from build123d import *

# Parameters (mm, degrees)
F0_R      = 38.1
F1_DEPTH  = 123.825
F2_R      = 6.35
F1_FACE_R = 31.75
F3_DEPTH  = 114.3
F4_R      = 4.292472


with BuildPart() as f1:
    # F0 (on Front) → F1 (new body)
    with BuildSketch(Plane.XZ):
        Circle(F0_R)
    extrude(amount=F1_DEPTH)

    # F2
    f2_edges = [f1.edges().sort_by_distance(p)[0] for p in [
        (-38.1, -123.825, 0),
    ]]
    fillet(f2_edges, radius=F2_R)

    # F1_face (on face) → F3 (cut)
    with BuildSketch(Plane.XZ.offset(123.825)):
        Circle(F1_FACE_R)
    extrude(amount=-F3_DEPTH, mode=Mode.SUBTRACT)

    # F4
    f4_edges = [f1.edges().sort_by_distance(p)[0] for p in [
        (-38.1, 0, 0),
    ]]
    fillet(f4_edges, radius=F4_R)


solid = f1.part
Read the model definition and answer for the solid it produces. Units are mm, in the model's axes. Coordinates: 2 decimals unless noted, no trailing zeros. Loops run counter-clockwise (first coordinate to the right, second up) from the corner with the lowest first, then second, coordinate; pieces in that order, holes last.
Q1. Each of these flat-tipped pins is pushed along its axis until it touches: pin 1 Ø6 at (x, y) = (-25, -68.5) entering from -Z; pin 2 Ø10 at (y, z) = (-68, -30) entering from -X; pin 3 Ø2 at (x, z) = (6.5, 7) entering from +Y; pin 4 Ø4 at (x, y) = (-1, -82.5) entering from +Z. Where does it stop, or does it pass through?
Q2. The part is cut by section B-B on z = 0. Write down the section's boundary in (x, y) (3 decimals).
Q3. The mould has two halves that part along Z. Classify faces 1 (the face through (-30.235, -60.091, -23.183)), 2 (the face through (-6.883, -67.475, -30.995)), 3 (the face through (0, 0, 0)): +Z half, -Z half, draft (parallel to the pull), parting line (faces both ways), or undercut.
Q4. Consider probe 1 along Z at (x, y) = (0, -38); probe 2 along Y at (x, z) = (-12.5, 1.5) (3 decimals); probe 3 along X at (y, z) = (-31.5, 27). Determine where each line is inside the solid, lowest interval first.
Q5. The part is cut by section A-A on x = 0. Write down the section's boundary in (y, z) (3 decimals), and give its area (3 significant figures).
Q6. The part is cut by section C-C on y = -44.5. Write down the section's boundary in (x, z), and give its area (3 significant figures).
Results below:
1. pin 1: stops at z = -31.11
1. pin 2: stops at x = -28.75
1. pin 3: stops at y = 0
1. pin 4: stops at z = 38.1
2. outline: (-38.1, -117.475) arc R6.35 ccw to (-31.75, -123.825) - (-31.75, -9.525) - (31.75, -9.525) - (31.75, -123.825) arc R6.35 ccw to (38.1, -117.475) - (38.1, -4.292) arc R4.292 ccw to (33.808, 0) - (-33.808, 0) arc R4.292 ccw to (-38.1, -4.292) - close
3. face 1: parting line
3. face 2: undercut
3. face 3: draft
4. probe 1: z = -38.1 to -31.75, 31.75 to 38.1
4. probe 2: y = -9.525 to 0
4. probe 3: x = -26.88 to -16.71, 16.71 to 26.88
5. outline: (-123.825, -31.75) arc R6.35 ccw to (-117.475, -38.1) - (-4.292, -38.1) arc R4.292 ccw to (0, -33.808) - (0, 33.808) arc R4.292 ccw to (-4.292, 38.1) - (-117.475, 38.1) arc R6.35 ccw to (-123.825, 31.75) - (-9.525, 31.75) - (-9.525, -31.75) - close
5. area: 2,150 mm2
6. outline: circle Ø76.2 at (0, 0); hole circle Ø63.5 at (0, 0)
6. area: 1,390 mm2
